Verification items for this drawing (mm, ordinates from the low corner). Round coordinates to 2 decimals unless told otherwise and drop trailing zeros. Order: outer loops, then holes, each group sorted by start corner. A loop starts at its lowest first (then second) coordinate and runs counter-clockwise, first axis right, second up. Notation, with made-up numbers: (-12.75, 3.5) -> (-6.75, 3.5) arc R30 ccw to (-6.75, 25.5) -> close; hole circle Ø10 at (-14.5, 19.5). An arc over 180 degrees is marked (long way). Answer in a Markdown table with one row per item. Add a question column.
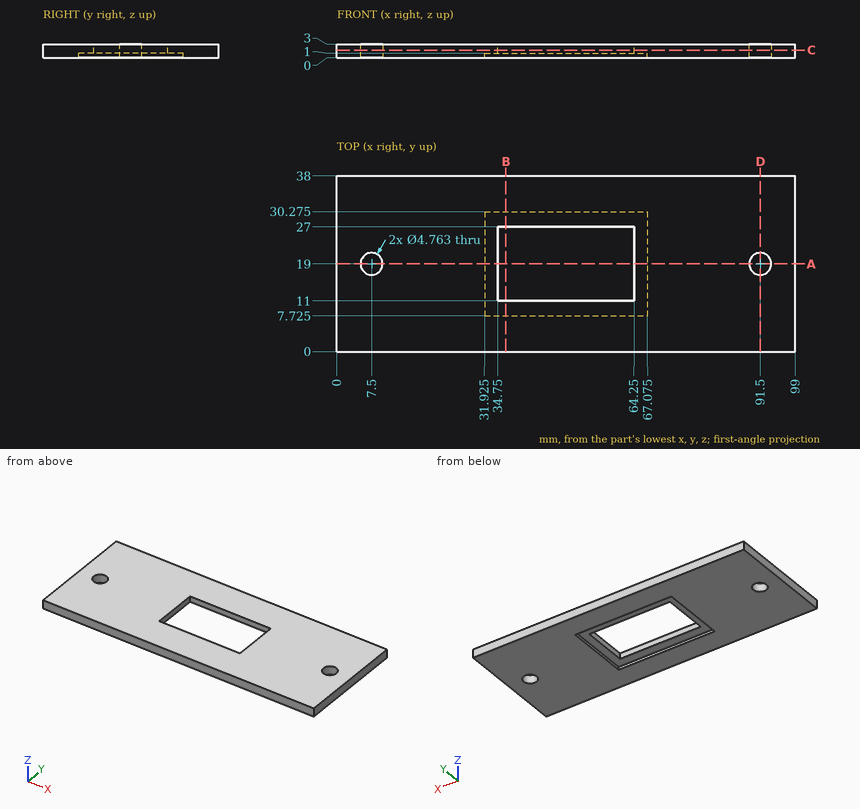
1) Cross-section at D-D, the plane x = 91.5. Record the boundary of the cut face in (y, z).
2) Cross-section at C-C, the plane z = 1.7. Record the boundary of the cut face in (x, y).
3) Cross-section at B-B, the plane x = 36.5. Record the boundary of the cut face in (y, z) (1 decimal).
4) Cross-section at A-A, the plane y = 19. Give the number of separate pieces and of enclosed holes in the cut face, and give its area (3 significant figures).
5) Thickness scan on L1, parallel to X at y = 21.5, z = 2.1; L2, parallel to Y at x = 91.5, z = 1.45; L3, parallel to Y at x = 59, z = 2.1. Record the ranges inside material, lowest first. Write a range as [from, to].
6) Depth check by flat-ended pin: P1, Ø8, axis at x = 45, y = 16, coming from the -Z side; P2, Ø11.5, axis at x = 47.5, y = 22.5, coming from the -Z side. Enter the tip coordinate at first touch or a pass-through.
Results below:
| question | item | result |
|---|---|---|
| 1 | outline | (0, 0) -> (16.62, 0) -> (16.62, 3) -> (0, 3) -> close; (21.38, 0) -> (38, 0) -> (38, 3) -> (21.38, 3) -> close |
| 2 | outline | (0, 0) -> (99, 0) -> (99, 38) -> (0, 38) -> close; hole circle Ø4.76 at (7.5, 19); hole (34.75, 11) -> (64.25, 11) -> (64.25, 27) -> (34.75, 27) -> close; hole circle Ø4.76 at (91.5, 19) |
| 3 | outline | (0, 0) -> (7.7, 0) -> (7.7, 1) -> (11, 1) -> (11, 3) -> (0, 3) -> close; (27, 1) -> (30.3, 1) -> (30.3, 0) -> (38, 0) -> (38, 3) -> (27, 3) -> close |
| 4 | separate pieces | 4 |
| 4 | enclosed holes | 0 |
| 4 | area | 174 mm² |
| 5 | L1 | [0, 34.75], [64.25, 99] |
| 5 | L2 | [0, 16.62], [21.38, 38] |
| 5 | L3 | [0, 11], [27, 38] |
| 6 | P1 | through |
| 6 | P2 | z = 1 |
